Design review of the part built by this model. Coordinates are the model's own, in mm. Face numbers are marked on the shaded views. A direction names the side the tool comes from. Round coordinates to 2 decimals unless told otherwise and drop trailing zeros. Loops run counter-clockwise (first coordinate to the right, second up) from the corner with the lowest first, then second, coordinate; pieces in that order, holes last. Notation, with made-up numbers: (-20, 23.25) - (26, 23.25) arc R30 ccw to (26, 58.25) - close; hole circle Ø4 at (3.25, -19). An arc over 180 degrees is marked (long way). Use one line per item in the form item = value. Start each with the question number.
(1) We need section C-C, the plane y = 10. Write out the cut boundary in (x, z), then the cut area to 3 significant figures.
(2) Machinability: for the marked faces 4, 5, 6 and 7, which of the approach directions +Z, -Z, +X, -X, +Y, -Y give a long, thin tool a straight path to every point of the face, cutting with its end or side? Answer none if there is none.
(3) We need section D-D, the plane x = 0. Give the number of separate pieces and of enclosed holes in the cut face, then the cut area to 3 significant figures.
(4) The part is to be moulded in two halves that separate along X. For the marked faces 1, 2 and 3, say which applies: released by +X, released by -X, zero draft, split by the parting line, or undercut.
(5) We need section A-A, the plane y = 33.4. Write out the cut boundary in (x, z), then the cut area to 3 significant figures.
(6) For pin 1 (5 mm diameter, centred on y = 31.5, z = -9.5, fed in from -X); pin 2 (5 mm diameter, centred on x = 6.5, z = -7, fed in from +Y); pin 3 (2.5 mm diameter, centred on x = -22.5, y = 19, fed in from +Z), all flat-tipped, find the tip position at first contact; note any pin that passes through.
(7) We need section B-B, the plane z = -8.5. Write out the cut boundary in (x, y).
(8) Wall thickness on probe 1 along X at (y, z) = (24.5, 0); probe 2 along Z at (x, y) = (17.5, 39); probe 3 along Z at (x, y) = (0, 24.5): over which ranges is each line inside the solid? List them lowest first. Write a range as [from, to].
from build123d import *

# Parameters (mm, degrees)
SKETCH_1_R          = 26
EXTRUDE_1_DEPTH     = 60.2
SKETCH_3_R          = 7
CUT_EXTRUDE_1_DEPTH = 30.1
SKETCH_4_R          = 21.5
CUT_EXTRUDE_2_DEPTH = 51
SKETCH_5_W          = 1.5
SKETCH_5_H          = 1.5
CUT_EXTRUDE_3_DEPTH = 50
SKETCH_9_W          = 5.5
SKETCH_9_H          = 24
CUT_EXTRUDE_4_DEPTH = 25
CUT_EXTRUDE_5_DEPTH = 2.1


with BuildPart() as part:
    # Эскиз1 → Бобышка-Вытянуть1 (new body)
    with BuildSketch(Plane(origin=(0, 0, 0), x_dir=(1, 0, 0), z_dir=(0, 1, 0))):
        with Locations(Location((0, 0, 0), (0, 0, 270))):
            Circle(SKETCH_1_R)
    extrude(amount=EXTRUDE_1_DEPTH)

    # Эскиз2 → Повернуть1 (revolve)
    with BuildSketch(Plane.XY):
        with BuildLine():
            Line((26, 60.2), (0, 60.2))
            Line((0, 60.2), (0, 63.5))
            ThreePointArc((0, 63.5), (13.10429319, 62.671703918), (26, 60.2))
        make_face()
    revolve(axis=Axis((0, 60.2, 0), (0, 1, 0)))

    # Эскиз3 → Вырез-Вытянуть1 (cut, symmetric)
    with BuildSketch(Plane.XY):
        with Locations((0, 33.4)):
            Circle(SKETCH_3_R)
        with BuildLine():
            Line((17.5, 0), (-17.5, 0))
            Line((-17.5, 0), (-17.5, 5))
            ThreePointArc((-17.5, 5), (-16.621320344, 7.121320344), (-14.5, 8))
            Line((-14.5, 8), (14.5, 8))
            ThreePointArc((14.5, 8), (16.621320344, 7.121320344), (17.5, 5))
            Line((17.5, 5), (17.5, 0))
        make_face()
    extrude(amount=CUT_EXTRUDE_1_DEPTH, both=True, mode=Mode.SUBTRACT)

    # Эскиз4 → Вырез-Вытянуть2 (cut)
    with BuildSketch(Plane(origin=(0, 0, 0), x_dir=(1, 0, 0), z_dir=(0, 1, 0))):
        with Locations(Location((0, 0, 0), (0, 0, 47.590982222))):
            Circle(SKETCH_4_R)
    extrude(amount=CUT_EXTRUDE_2_DEPTH, mode=Mode.SUBTRACT)

    # Эскиз5 → Вырез-Повернуть1 (revolve, cut)
    with BuildSketch(Plane.XY, mode=Mode.PRIVATE) as cut_revolve_1_sk:
        with Locations((-25.25, 56.45)):
            Rectangle(SKETCH_5_W, SKETCH_5_H)
        with Locations((-25.25, 53.95)):
            Rectangle(SKETCH_5_W, SKETCH_5_H)
    revolve(cut_revolve_1_sk.sketch.rotate(Axis((0, 37.032198444, 0), (0, 1, 0)), 270), axis=Axis((0, 37.032198444, 0), (0, 1, 0)), mode=Mode.SUBTRACT)

    # Эскиз6 → Вырез-Вытянуть3 (cut)
    with BuildSketch(Plane(origin=(0, 0, 0), x_dir=(0, 0, -1), z_dir=(1, 0, 0))):
        with BuildLine():
            Line((-4, 6), (-4, 25))
            ThreePointArc((-4, 25), (-4.878679656, 27.121320344), (-7, 28))
            Line((-7, 28), (-10, 28))
            ThreePointArc((-10, 28), (-12.121320344, 27.121320344), (-13, 25))
            Line((-13, 25), (-13, 6))
            ThreePointArc((-13, 6), (-12.121320344, 3.878679656), (-10, 3))
            Line((-10, 3), (-7, 3))
            ThreePointArc((-7, 3), (-4.878679656, 3.878679656), (-4, 6))
        make_face()
        with BuildLine():
            Line((10, 3), (7, 3))
            ThreePointArc((7, 3), (4.878679656, 3.878679656), (4, 6))
            Line((4, 6), (4, 25))
            ThreePointArc((4, 25), (4.878679656, 27.121320344), (7, 28))
            Line((7, 28), (10, 28))
            ThreePointArc((10, 28), (12.121320344, 27.121320344), (13, 25))
            Line((13, 25), (13, 6))
            ThreePointArc((13, 6), (12.121320344, 3.878679656), (10, 3))
        make_face()
    extrude(amount=-CUT_EXTRUDE_3_DEPTH, mode=Mode.SUBTRACT)

    # Эскиз9 → Вырез-Вытянуть4 (cut, symmetric)
    with BuildSketch(Plane(origin=(0, 0, 0), x_dir=(0, 0, -1), z_dir=(1, 0, 0))):
        with Locations((-26.254259625, 33.4)):
            Rectangle(SKETCH_9_W, SKETCH_9_H)
        with Locations((26.254259625, 33.4)):
            Rectangle(SKETCH_9_W, SKETCH_9_H)
    extrude(amount=CUT_EXTRUDE_4_DEPTH, both=True, mode=Mode.SUBTRACT)

    # Эскиз10 → Вырез-Вытянуть5 (cut)
    with BuildSketch(Plane(origin=(0, 63, 0), x_dir=(1, 0, 0), z_dir=(0, 1, 0))):
        Polygon((22.641485295, 0), (21.227271732, 1.414213562), (20.727271732, 1.414213562), (21.891485295, 0.25), (18.141485295, 0.25), (18.141485295, -0.25), (21.891485295, -0.25), (20.727271732, -1.414213562), (21.227271732, -1.414213562), align=None)
    extrude(amount=-CUT_EXTRUDE_5_DEPTH, mode=Mode.SUBTRACT)


solid = part.part
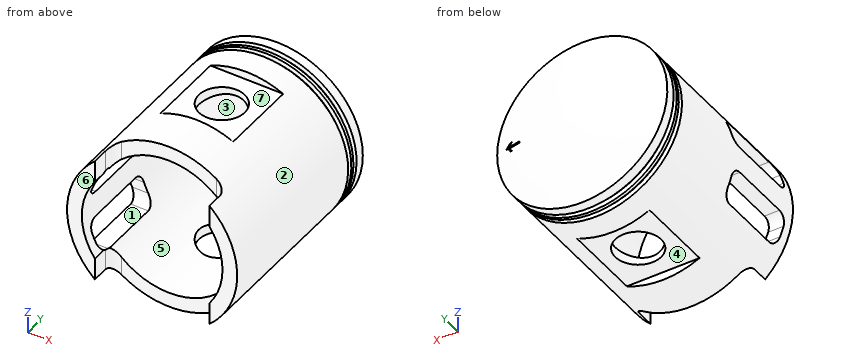
Data:
q1.outline = (-25.69, -4) - (-21.12, -4) arc R21.5 cw to (-21.12, 4) - (-25.69, 4) arc R26 ccw to start; (-22.52, -13) arc R26 ccw (long way) to (-22.52, 13) - (-17.12, 13) arc R21.5 cw (long way) to (-17.12, -13) - close
q1.area = 584 mm^2
q2.face_4 = -Z, +X, -X
q2.face_5 = -Y
q2.face_6 = +Z, -Z, +X, -X, -Y
q2.face_7 = +Z, +X, -X
q3.separate_pieces = 3
q3.enclosed_holes = 0
q3.area = 795 mm^2
q4.face_1 = zero draft
q4.face_2 = split by the parting line
q4.face_3 = undercut
q5.outline = (-11.12, -23.5) - (-7, -23.5) - (-7, -20.33) arc R21.5 cw to (-7, 20.33) - (-7, 23.5) - (-11.12, 23.5) arc R26 ccw to start; (7, -23.5) - (11.12, -23.5) arc R26 ccw to (11.12, 23.5) - (7, 23.5) - (7, 20.33) arc R21.5 cw to (7, -20.33) - close
q5.area = 530 mm^2
q6.pin_1 = -25.04
q6.pin_2 = 63.26
q6.pin_3 = 14.98
q7.outline = (-24.57, 0) - (-19.75, 0) - (-19.75, 3) - (-24.57, 3) - close; (-24.57, 28) - (-19.75, 28) - (-19.75, 51) - (19.75, 51) - (19.75, 0) - (24.57, 0) - (24.57, 53.2) - (22.98, 53.2) - (22.98, 54.7) - (24.57, 54.7) - (24.57, 55.7) - (22.98, 55.7) - (22.98, 57.2) - (24.57, 57.2) - (24.57, 60.2) arc R103.73 ccw to (-24.57, 60.2) - (-24.57, 57.2) - (-22.98, 57.2) - (-22.98, 55.7) - (-24.57, 55.7) - (-24.57, 54.7) - (-22.98, 54.7) - (-22.98, 53.2) - (-24.57, 53.2) - close
q8.probe_1 = [-26, -21.5], [21.5, 26]
q8.probe_2 = [-19.23, -12.49], [12.49, 19.23]
q8.probe_3 = [-23.5, -21.5], [21.5, 23.5]
